Could you check a few things on this model? Use its own coordinates, in mm. A direction names the side the tool comes from. Round coordinates to 2 decimals unless told otherwise and drop trailing zeros. Loops run counter-clockwise (first coordinate to the right, second up) from the corner with the lowest first, then second, coordinate; pieces in that order, holes last. Notation, with made-up numbers: (39.25, 45) -> (82.25, 45) arc R22 cw to (82.25, 83) -> close; hole circle Ø4 at (-31, -18.5). An arc over 180 degrees is marked (long way). Write each question's results on one line, items separated by ' | '. Start each with the question number.
1) For P1, Ø2, axis at x = -257.5, z = 0.5, coming from the +Y side, with a flat end and sliding along its axis, tell me the tip position at first contact or that it passes through.
2) Which directions (+Z, -Z, +X, -X, +Y, -Y) give clear straight access to the entire face, cutting with the end or side of a thin tool? Please do faces 1 (the cylindrical face through (-279.67, -654.86, 1.97)), 2 (the flat face through (-246.92, -610, 2)), 3 (the flat face through (-265, -600, 4)).
3) Imagine slicing it at A-A, the plane z = 1.15. List the corners of the cut face in (x, y) for me (3 decimals).
4) We'd pull the mould along X, two halves only. Please class faces 4 (the flat face through (-245.09, -549.96, 1.97)), 5 (the flat face through (-286.92, -628, 2)), 6 (the cylindrical face through (-258.446, -548.831, 1.972)): pulls with the +X half, pulls with the -X half, needs draft (parallel to the pull), parting line crosses it, or undercut.
5) If I drill on probe 1 along Y at (x, z) = (-275, 1.1); probe 2 along Y at (x, z) = (-257.5, 3.15); probe 3 along Y at (x, z) = (-279, 1.3), over which ranges is the centre line in solid material (lowest first)?
6) Imagine slicing it at C-C, the plane x = -281.5. List the corners of the cut face in (y, z) for me.
7) Imagine slicing it at B-B, the plane y = -594.5. List the corners of the cut face in (x, z) for me.
from build123d import *

# Parameters (mm, degrees)
BOSS_EXTRUDE1_DEPTH = 4


with BuildPart() as part:
    # Sketch2 → Boss-Extrude1 (new body)
    with BuildSketch(Plane.XY):
        Polygon((-243.202124872, -545.912292309), (-261.32800293, -537.460021973), (-286.920013428, -592.342041016), (-286.920013428, -665.044006348), (-246.92041444, -665.044006348), (-246.92041444, -553.886157392), align=None)
        with BuildLine():
            ThreePointArc((-256.682006836, -652.315040871), (-259.638579462, -654.80647695), (-257.159011841, -657.773010254))
            ThreePointArc((-257.159011841, -657.773010254), (-254.180566252, -655.283485786), (-256.682006836, -652.315040871))
        make_face(mode=Mode.SUBTRACT)
        with BuildLine():
            ThreePointArc((-276.920013428, -652.294006348), (-279.672667512, -654.918648036), (-277.159011841, -657.773010254))
            ThreePointArc((-277.159011841, -657.773010254), (-274.171775379, -655.158601231), (-276.920013428, -652.294006348))
        make_face(mode=Mode.SUBTRACT)
        with BuildLine():
            ThreePointArc((-276.136016846, -602.418029785), (-279.582956118, -604.374783929), (-277.476013184, -607.732025146))
            ThreePointArc((-277.476013184, -607.732025146), (-274.263780083, -605.716086644), (-276.136016846, -602.418029785))
        make_face(mode=Mode.SUBTRACT)
        with BuildLine():
            ThreePointArc((-256.682006836, -602.315002441), (-259.662954971, -604.8043291), (-257.159011841, -607.773010254))
            ThreePointArc((-257.159011841, -607.773010254), (-254.180547037, -605.283466564), (-256.682006836, -602.315002441))
        make_face(mode=Mode.SUBTRACT)
        with BuildLine():
            ThreePointArc((-265.17401123, -566.142028809), (-267.635869624, -569.341884059), (-264.25201416, -571.544006348))
            ThreePointArc((-264.25201416, -571.544006348), (-262.235793714, -568.420211554), (-265.17401123, -566.142028809))
        make_face(mode=Mode.SUBTRACT)
        with BuildLine():
            ThreePointArc((-254.228012085, -549.178039551), (-258.493761484, -548.880446167), (-257.878021241, -553.111999511))
            ThreePointArc((-257.878021241, -553.111999511), (-254.467220991, -552.616353449), (-254.228012085, -549.178039551))
        make_face(mode=Mode.SUBTRACT)
    extrude(amount=BOSS_EXTRUDE1_DEPTH)


solid = part.part
Checked values:
1) P1: y = -538.78
2) face 1: +Z, -Z | face 2: +Z, -Z, +X, -Y | face 3: +Z, +X, -X, +Y, -Y
3) outline: (-286.92, -665.044) -> (-246.92, -665.044) -> (-246.92, -553.886) -> (-243.202, -545.912) -> (-261.328, -537.46) -> (-286.92, -592.342) -> close; hole circle Ø5.486 at (-276.923, -605.045); hole (-277.159, -657.773) arc R2.745 ccw (long way) to (-276.92, -652.294) arc R2.744 ccw to start; hole (-265.174, -566.142) arc R2.749 ccw (long way) to (-264.252, -571.544) arc R2.75 ccw to start; hole circle Ø5.479 at (-256.91, -655.045); hole (-257.878, -553.112) arc R2.746 ccw to (-254.228, -549.178) arc R2.746 ccw (long way) to start; hole (-257.159, -607.773) arc R2.739 ccw (long way) to (-256.682, -602.315) arc R2.739 ccw (long way) to start
4) face 4: pulls with the +X half | face 5: pulls with the -X half | face 6: undercut
5) probe 1: -665.04 to -657.01, -653.07 to -607, -603.09 to -566.78 | probe 2: -665.04 to -657.72, -652.37 to -607.72, -602.36 to -553.3, -548.2 to -539.25 | probe 3: -665.04 to -656.84, -653.24 to -606.84, -603.25 to -575.36
6) outline: (-665.04, 0) -> (-580.72, 0) -> (-580.72, 4) -> (-665.04, 4) -> close
7) outline: (-286.92, 0) -> (-246.92, 0) -> (-246.92, 4) -> (-286.92, 4) -> close
